from build123d import *

# Parameters (mm, degrees)
F0_W     = 20
F0_H     = 15
F1_DEPTH = 7
F3_W     = 10.6
F3_H     = 10.6
F4_DEPTH = 3.6
F5_R     = 2.2
F6_DEPTH = 7


with BuildPart() as f1:
    # F0 (on Top) → F1 (new body)
    with BuildSketch(Plane.XY):
        Rectangle(F0_W, F0_H)
    extrude(amount=F1_DEPTH)

    # F3 (on offset) → F4 (cut)
    with BuildSketch(Plane.XY.offset(2)):
        with Locations((-5, 0)):
            Rectangle(F3_W, F3_H)
    extrude(amount=F4_DEPTH, mode=Mode.SUBTRACT)

    # F5 (on Top) → F6 (join, through all)
    with BuildSketch(Plane.XY):
        with Locations((-5, 0)):
            Circle(F5_R)
    extrude(amount=F6_DEPTH)


solid = f1.part
Verification items for the finished model (mm, model axes). A direction names the side the tool comes from. Coordinates: 2 decimals unless noted, no trailing zeros. Loops run counter-clockwise (first coordinate to the right, second up) from the corner with the lowest first, then second, coordinate; pieces in that order, holes last. Notation, with made-up numbers: (54, -2) -> (95, -2) arc R9 ccw to (95, 6) -> close; hole circle Ø2 at (-17, -4.5). An arc over 180 degrees is marked (long way). Answer as CSV lines item,"result".
1) Cross-section at C-C, the plane y = 0. Record the cut outline in (x, z).
Found:
outline,"(-10, 0) -> (10, 0) -> (10, 7) -> (-10, 7) -> (-10, 5.6) -> (-7.2, 5.6) -> (-7.2, 2) -> (-10, 2) -> close; hole (-2.8, 2) -> (0.3, 2) -> (0.3, 5.6) -> (-2.8, 5.6) -> close"
2) Cross-section at B-B, the plane z = 4. Record the cut outline in (x, y).
Found:
outline,"(-10, -7.5) -> (10, -7.5) -> (10, 7.5) -> (-10, 7.5) -> (-10, 5.3) -> (0.3, 5.3) -> (0.3, -5.3) -> (-10, -5.3) -> close; circle Ø4.4 at (-5, 0)"
3) Release check for a two-part mould opening along Z. For faces 1 (the flat face through (-10, 0, 1)), 2 (the flat face through (0, 0, 7)), 3 (the flat face through (-2.6, 0.1, 2)) record: +Z half, -Z half, draft (parallel to the pull), parting line (faces both ways), or undercut.
Found:
face 1,"draft"
face 2,"+Z half"
face 3,"undercut"
4) Cross-section at A-A, the plane x = -2.5. Record the cut outline in (y, z), then the cut area to 3 significant figures.
Found:
outline,"(-7.5, 0) -> (7.5, 0) -> (7.5, 7) -> (-7.5, 7) -> close; hole (-5.3, 2) -> (5.3, 2) -> (5.3, 5.6) -> (-5.3, 5.6) -> close"
area,"66.8 mm2"
5) Thickness scan on L1, parallel to Z at x = -1.75, y = -3; L2, parallel to Y at x = -6.75, z = 2.75; L3, parallel to Y at x = -4.25, z = 2.5. Record the ranges inside material, lowest first. Write a range as from..to.
Found:
L1,"z = 0..2, 5.6..7"
L2,"y = -7.5..-5.3, -1.33..1.33, 5.3..7.5"
L3,"y = -7.5..-5.3, -2.07..2.07, 5.3..7.5"
6) Tool access check on faces 4 (the flat face through (-5, 5.3, 4)), 5 (the flat face through (0, 7.5, 3)), 6 (the flat face through (-2.6, 0.1, 5.6)). Record the directions out of +Z, -Z, +X, -X, +Y, -Y that give a thin tool (end or side, any length) a straight path to the whole face; none if there is none.
Found:
face 4,"-X"
face 5,"+Z, -Z, +X, -X, +Y"
face 6,"none"
7) Cross-section at D-D, the plane x = -5. Record the cut outline in (y, z).
Found:
outline,"(-7.5, 0) -> (7.5, 0) -> (7.5, 7) -> (-7.5, 7) -> close; hole (-5.3, 2) -> (-2.2, 2) -> (-2.2, 5.6) -> (-5.3, 5.6) -> close; hole (2.2, 2) -> (5.3, 2) -> (5.3, 5.6) -> (2.2, 5.6) -> close"
